For this review, take the finished solid that the model builds, in its own axes (mm). Give positions to 0.01 mm unless a question says otherwise; leave off trailing zeros. Order: outer loops, then holes, each group sorted by start corner. A loop starts at its lowest first (then second) coordinate and runs counter-clockwise, first axis right, second up. Notation, with made-up numbers: (56.25, 19.25) -> (81.25, 19.25) arc R25 cw to (81.25, 41.25) -> close; hole circle Ø3 at (10, 76). An arc over 180 degrees is marked (long way). Return JSON: item names as keys, results as strings. Group by question number.
1) Insertion check: P1, Ø5, axis at x = 265.5, y = -47, coming from the -Z side; P2, Ø1, axis at y = -31, z = 127.5, coming from the +X side; P3, Ø2.5, axis at x = 239.5, z = 101.5, coming from the +Y side; P4, Ø12, axis at x = -203, z = 104, coming from the +Y side. Each pin has a flat end and moves straight along its axis. Give the tip position at first contact, or say it passes through.
2) Add section A-A (y = 27). Give the boundary of the cut face in (x, z), then the cut area to 3 significant figures.
3) To check wall thickness, follow line 1 along X through (y, z) = (36.5, 102.5); line 2 along Z through (x, y) = (237, 26); line 3 along Y through (x, z) = (156.5, 15.5). State the ranges of each line that lie inside material, in increasing order.
4) Add section B-B (x = -209). Give the boundary of the cut face in (y, z), then the cut area to 3 significant figures.
Autodesk Inventor part; units mm, degrees
ref_plane "Work Plane1" through (0, 60, 0) normal (0, 1, 0) x (-1, 0, 0)
ref_plane "YZ Plane" through (0, 0, 0) normal (1, 0, 0) x (0, 1, 0)
ref_plane "XY Plane" through (0, 0, 0) normal (0, 0, 1) x (1, 0, 0)
sketch "Sketch1" plane through (0, 0, 0) normal (0, 0, 1) x (1, 0, 0)
  line L0 (-337.5, 75) -> (337.5, 75)
  line L1 (337.5, 75) -> (337.5, -75)
  line L2 (337.5, -75) -> (-337.5, -75)
  line L3 (-337.5, -75) -> (-337.5, 75)
  line L4 (-337.5, 75) -> (337.5, -75) construction
  line L5 (337.5, 75) -> (-337.5, -75) construction
  point P0 (0, 0)
  dimension "d0" = 675
  dimension "d1" = 150
extrude "Extrusion1" add sketch "Sketch1" along normal blind 150
sketch "Sketch2" plane through (0, 0, 150) normal (0, 0, 1) x (1, 0, 0)
  line L0 (-400, 225) -> (400, 225)
  line L1 (400, 225) -> (400, -225)
  line L2 (400, -225) -> (-400, -225)
  line L3 (-400, -225) -> (-400, 225)
  line L4 (-337.5, 0) -> (-187.5, 0)
  line L5 (-337.5, 0) -> (-337.5, 40)
  line L6 (-337.5, 0) -> (-337.5, -40)
  line L7 (337.5, 0) -> (287.5, 0)
  line L8 (337.5, 0) -> (337.5, 40)
  line L9 (337.5, 0) -> (337.5, -40)
  arc A0 (-187.5, 75) -> (-337.5, 40) centre (-150.241, -423.6098) ccw
  line L10 (-187.5, 75) -> (287.5, 75)
  arc A1 (337.5, 40) -> (287.5, 75) centre (273.2116, 1.3736) ccw
  arc A2 (-337.5, -40) -> (-187.5, -75) centre (-150.241, 423.6098) ccw
  line L11 (-187.5, -75) -> (287.5, -75)
  arc A3 (287.5, -75) -> (337.5, -40) centre (273.2116, -1.3736) ccw
  point P0 (0, 0)
  dimension "d4" = 800
  dimension "d5" = 450
  dimension "d14" = 50
  dimension "d15" = 40
  dimension "d16" = 40
  dimension "d17" = 500
  dimension "d18" = 75
extrude "Extrusion2" cut sketch "Sketch2" against normal blind 150
sketch "Sketch3" plane through (-187.5, 75, 0) normal (0, 1, 0) x (1, 0, 0)
  line L0 (-312.5, 400) -> (687.5, 400)
  line L1 (687.5, 400) -> (687.5, -400)
  line L2 (687.5, -400) -> (-312.5, -400)
  line L3 (-312.5, -400) -> (-312.5, 400)
  line L4 (525, 0) -> (525, -150)
  line L5 (525, -75) -> (475, -75)
  line L6 (-150, -150) -> (-150, 0)
  line L7 (-150, -75) -> (-150, -35)
  line L8 (0, 0) -> (475, 0)
  arc A0 (0, 0) -> (-150, -35) centre (37.259, -498.6098) ccw
  line L9 (525, -75) -> (525, -35)
  line L10 (525, 0) -> (475, 0)
  arc A1 (525, -35) -> (475, 0) centre (460.7116, -73.6264) ccw
  line L11 (-150, -75) -> (-150, -115)
  arc A2 (-150, -115) -> (0, -150) centre (37.259, 348.6098) ccw
  line L12 (525, -75) -> (525, -115)
  arc A3 (475, -150) -> (525, -115) centre (460.7116, -76.3736) ccw
  line L13 (475, -150) -> (0, -150)
  line L14 (0, -150) -> (475, -150)
  point P0 (187.5, 0)
  dimension "d23" = 40
  dimension "d24" = 500
  dimension "d25" = 40
  dimension "d26" = 75
extrude "Extrusion3" cut sketch "Sketch3" against normal blind 150 contours L0 L1 L2 L3 | L4 A1 L10
sketch "Sketch4" plane through (0, 0, 150) normal (0, 0, 1) x (1, 0, 0)
  spline S0 degree 4 poles (287.5, 72) (275.7106, 75.6696) (272.2633, 78.0977) (241.0041, 87.3899) (212.1922, 94.1056) (186.8012, 99.4436) (162.2405, 102.6617) (136.499, 103.3609) (115.3024, 103.9082) (87.5125, 99.0497) (77.8593, 96.7101) (62.5936, 91.6603) (56.4872, 88.8369) (50.2371, 85.9481) (43.0983, 79.8721) (41.263, 78.3038) (35.0709, 71.8313) (41.0621, 66.1136) (43.5349, 66.5804) (51.0426, 65.1949) (57.2037, 65.9223) (63.437, 66.335) (78.7454, 67.9836) (88.3716, 68.7088) (116.236, 70.8678) (137.1854, 71.569) (162.8258, 72.2403) (187.1936, 73.1117) (212.5281, 72.7462) (241.0177, 72.4966) (272.1667, 71.6209) (275.8592, 71.8531) (287.5, 71.2) knots 0 0 0 0 0 0.082908 0.121264 0.162409 0.203325 0.244067 0.284728 0.322462 0.357388 0.387441 0.412707 0.436373 0.45684 0.477222 0.496964 0.514702 0.533384 0.551956 0.570848 0.593257 0.617753 0.647324 0.681959 0.719554 0.76011 0.800663 0.841217 0.881776 0.91937 1 1 1 1 1
  arc A0 (287.5, 71.2) -> (287.5, 72) centre (286.5835, 71.6) ccw
  point P0 (0, 0)
  point P1 (274.89, 76.355)
  point P2 (262.2875, 80.71)
  point P3 (237.1175, 87.97)
  point P4 (211.975, 94.0325)
  point P5 (186.8575, 99.02)
  point P6 (161.785, 102.1575)
  point P7 (136.7575, 103.3225)
  point P8 (111.775, 102.5875)
  point P9 (86.8675, 98.68)
  point P10 (74.4425, 95.465)
  point P11 (62.0425, 91.2)
  point P12 (55.855, 88.53)
  point P13 (49.685, 85.06)
  point P14 (43.5475, 80.2425)
  point P15 (40.49, 77.395)
  point P16 (37.5, 71.6)
  point P17 (40.73, 67.15)
  point P18 (43.875, 66.3)
  point P19 (50.14, 65.645)
  point P20 (56.385, 65.7925)
  point P21 (62.6225, 66.3375)
  point P22 (75.095, 67.555)
  point P23 (87.57, 68.6475)
  point P24 (112.5275, 70.43)
  point P25 (137.5025, 71.54)
  point P26 (162.485, 72.275)
  point P27 (187.47, 72.86)
  point P28 (212.4725, 72.77)
  point P29 (237.48, 72.43)
  point P30 (262.4925, 71.94)
  point P31 (274.9975, 71.7075)
  point P32 (287.5, 75)
  dimension "d31" = 1
extrude "Extrusion4" cut sketch "Sketch4" against normal blind 150
sketch "Sketch5" plane through (0, 0, 150) normal (0, 0, 1) x (1, 0, 0)
  spline S0 degree 4 poles (278.5919, 75) (280.4602, 74.3245) (282.4435, 73.6259) (284.707, 72.8694) (287.5, 72) knots 0 0 0 0 0 1 1 1 1 1
  line L0 (287.5, 72) -> (287.5, 75)
  line L1 (287.5, 75) -> (278.5919, 75)
  point P0 (0, 0)
extrude "Extrusion5" cut sketch "Sketch5" against normal blind 150
sketch "Sketch8" plane through (0, 0, 150) normal (0, 0, 1) x (1, 0, 0)
  line L0 (38.5386, 75) -> (-187.5, 75)
  line L1 (-187.5, 75) -> (-187.5, -75)
  line L2 (-187.5, -75) -> (287.5, -75)
  line L3 (287.5, -75) -> (287.5, 71.2)
  arc A0 (-337.5, -40) -> (-187.5, -75) centre (-150.241, 423.6098) ccw
  line L4 (-187.5, 75) -> (-187.5, -75)
  arc A1 (-187.5, 75) -> (-337.5, 40) centre (-150.241, -423.6098) ccw
  line L5 (-337.5, -40) -> (-337.5, 40)
  line L6 (287.5, -75) -> (287.5, 71.2)
  arc A2 (287.5, -75) -> (337.5, -40) centre (273.2116, -1.3736) ccw
  line L7 (337.5, 40) -> (337.5, -40)
  arc A3 (337.5, 40) -> (287.5, 75) centre (273.2116, 1.3736) ccw
  line L8 (287.5, 72) -> (287.5, 75)
  point P0 (0, 0)
sketch "Sketch9" plane through (-187.5, 75, 150) normal (0, 1, 0) x (1, 0, 0)
  point P0 (187.5, 150)
sketch "Sketch10" plane through (-337.5, -40, 115) normal (-1, 0, 0) x (0, 0, 1)
  line L0 (0, 0) -> (0, 80)
  line L1 (0, 80) -> (-80, 80)
  line L2 (-80, 80) -> (-80, 0)
  line L3 (-80, 0) -> (0, 0)
  point P0 (-115, 40)
ref_plane "Work Plane1" through (0, 60, 0) normal (0, 1, 0) x (-1, 0, 0)
sketch "Sketch11" plane through (0, 60, 0) normal (0, 1, 0) x (-1, 0, 0)
  line L0 (-287.5, 0) -> (-287.5, 150)
  line L1 (-287.5, 75) -> (-287.5, 47.5)
  line L2 (-287.5, 47.5) -> (-237.5, 47.5)
  circle A0 centre (-237.5, 47.5) radius 4
  line L3 (-287.5, 75) -> (-187.5, 75)
  line L4 (-287.5, 47.5) -> (-87.5, 47.5)
  circle A1 centre (-87.5, 47.5) radius 4
  circle A2 centre (-237.5, 102.5) radius 4
  circle A3 centre (-87.5, 102.5) radius 4
  point P0 (0, 0)
  dimension "d70" = 27.5
  dimension "d71" = 50
  dimension "d72" = 8
  dimension "d73" = 100
  dimension "d74" = 200
  dimension "d75" = 8
extrude "Extrusion8" cut sketch "Sketch11" against normal mid plane 100
Evaluation:
{
 "1": {"P1": "z = 0", "P2": "x = 328.55", "P3": "y = 10", "P4": "y = 74.2"},
 "2": {"outline": "(-337.5, 35) arc R500 ccw to (-187.5, 0) -> (287.5, 0) arc R75 ccw to (337.5, 35) -> (337.5, 115) arc R75 ccw to (287.5, 150) -> (-187.5, 150) arc R500 ccw to (-337.5, 115) -> close; hole circle Ø8 at (87.5, 47.5); hole circle Ø8 at (87.5, 102.5); hole circle Ø8 at (237.5, 47.5); hole circle Ø8 at (237.5, 102.5)", "area": "95,800 mm^2"},
 "3": {"line 1": "-337.5 to 83.5, 91.5 to 233.5, 241.5 to 337.5", "line 2": "0 to 43.53, 51.47 to 98.53, 106.47 to 150", "line 3": "-75 to 72.1"},
 "4": {"outline": "(-72.93, 2.07) -> (72.93, 2.07) -> (72.93, 147.93) -> (-72.93, 147.93) -> close", "area": "21,300 mm^2"}
}
